The drawing under review shows one solid part. Ordinate dimensions are in mm from its lowest x, y, z. A direction names the side the tool comes from. Coordinates: 2 decimals unless noted, no trailing zeros. Write each loop counter-clockwise with the first axis right and the second up, starting at its lowest first coordinate (ties: lowest second). Pieces come first, ordered by that corner, then holes.
Q1. Clearance check with flat-ended pins moving along their axes: pin 1 Ø3 at (y, z) = (49, 5.5) entering from +X; pin 2 Ø1.4 at (x, z) = (3.5, 6) entering from +Y; pin 3 Ø4 at (y, z) = (46.5, 2.5) entering from -X; pin 4 Ø1 at (y, z) = (20.5, 7.5) entering from +X. State where each tip first meets the part, or that it passes through.
Q2. Machinability: for the marked faces 4 and 5, which of the approach directions +Z, -Z, +X, -X, +Y, -Y give a long, thin tool a straight path to every point of the face, cutting with its end or side? Answer none if there is none.
Q3. Add section A-A, the plane x = 6.25. Give the boundary of the cut face in (y, z) (1 decimal), plus the area to 3 significant figures.
Q4. Add section C-C, the plane z = 1. Give the boundary of the cut face in (x, y) (1 decimal).
Q5. The part is to be moulded in two halves that separate along Z. For the marked faces 1, 2 and 3, say which applies: +Z half, -Z half, draft (parallel to the pull), parting line (faces both ways), or undercut.
Q6. Add section D-D, the plane x = 9.75. Give the boundary of the cut face in (y, z) (1 decimal), plus the area to 3 significant figures.
Q7. Add section B-B, the plane y = 44.5. Give the boundary of the cut face in (x, z) (1 decimal).
Q8. To check wall thickness, follow probe 1 along Y at (x, z) = (5.5, 9.25) (1 decimal); probe 2 along Y at (x, z) = (6.25, 5.5); probe 3 along Z at (x, y) = (2.5, 44) (1 decimal). State the ranges of each line that lie inside material, in increasing order.
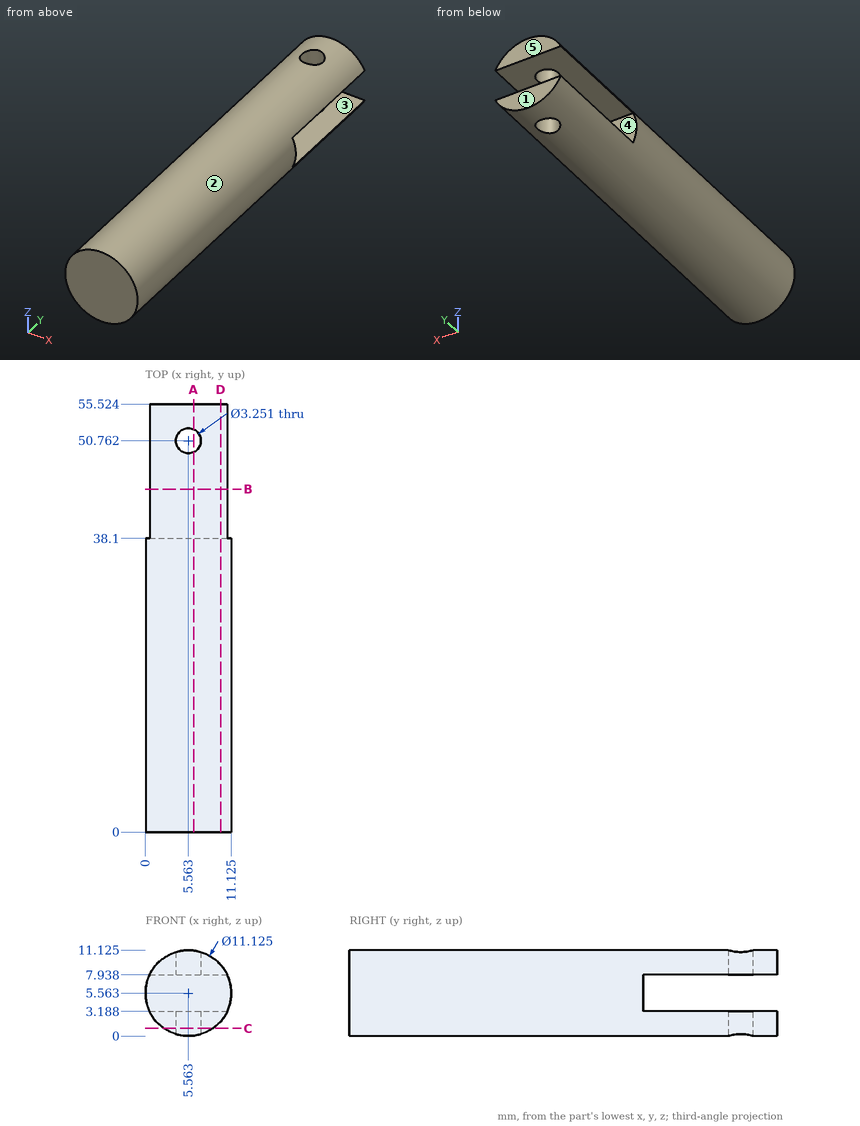
Here are the results:
1. pin 1: passes through
1. pin 2: stops at y = 38.1
1. pin 3: stops at x = 0.53
1. pin 4: stops at x = 10.94
2. face 4: +X, -X, +Y
2. face 5: +Z, -Z, +X, -X, +Y
3. outline: (0, 0) - (49.3, 0) - (49.3, 3.2) - (38.1, 3.2) - (38.1, 7.9) - (49.3, 7.9) - (49.3, 11.1) - (0, 11.1) - close; (52.2, 0) - (55.5, 0) - (55.5, 3.2) - (52.2, 3.2) - close; (52.2, 7.9) - (55.5, 7.9) - (55.5, 11.1) - (52.2, 11.1) - close
3. area: 512 mm2
4. outline: (2.4, 0) - (8.7, 0) - (8.7, 55.5) - (2.4, 55.5) - close; hole circle Ø3.3 at (5.6, 50.8)
5. face 1: draft
5. face 2: parting line
5. face 3: undercut
6. outline: (0, 1.9) - (55.5, 1.9) - (55.5, 3.2) - (38.1, 3.2) - (38.1, 7.9) - (55.5, 7.9) - (55.5, 9.2) - (0, 9.2) - close
6. area: 324 mm2
7. outline: (0.5, 3.2) arc R5.6 ccw to (10.6, 3.2) - close; (0.5, 7.9) - (10.6, 7.9) arc R5.6 ccw to start
8. probe 1: y = 0 to 49.1, 52.4 to 55.5
8. probe 2: y = 0 to 38.1
8. probe 3: z = 0.9 to 3.2, 7.9 to 10.2
